Verification items for this drawing (mm, ordinates from the low corner). A direction names the side the tool comes from. Coordinates: 2 decimals unless noted, no trailing zeros. Order: outer loops, then holes, each group sorted by start corner. A loop starts at its lowest first (then second) coordinate and runs counter-clockwise, first axis right, second up. Notation, with made-up numbers: (82.25, 69) - (89.25, 69) arc R13 ccw to (89.25, 79) - close; hole circle Ø3 at (77, 8.5). An arc over 180 degrees is marked (long way). Use CSV: the item, a comma, the result in double quotes. Start each with the question number.
1) Tool access check on the marked faces 1 and 2. Record the directions out of +Z, -Z, +X, -X, +Y, -Y that give a thin tool (end or side, any length) a straight path to the whole face; none if there is none.
2) Sectioned sample at B-B, the plane x = 21. Record the cut outline in (y, z).
3) Thickness scan on probe 1 along X at (y, z) = (15.25, 4.5); probe 2 along Z at (x, y) = (17.75, 9.25); probe 3 along Z at (x, y) = (22.25, 10). Record the ranges inside material, lowest first. Write a range as [from, to].
4) Depth check by flat-ended pin: P1, Ø1.5, axis at x = 11, z = 4.5, coming from the +Y side; P2, Ø6, axis at x = 23.5, y = 15.5, coming from the +Z side; P3, Ø1, axis at y = 2, z = 8.5, coming from the +X side. Enter the tip coordinate at first touch or a pass-through.
5) Sectioned sample at A-A, the plane x = 5. Record the cut outline in (y, z) (1 decimal), and give its area (3 significant figures).
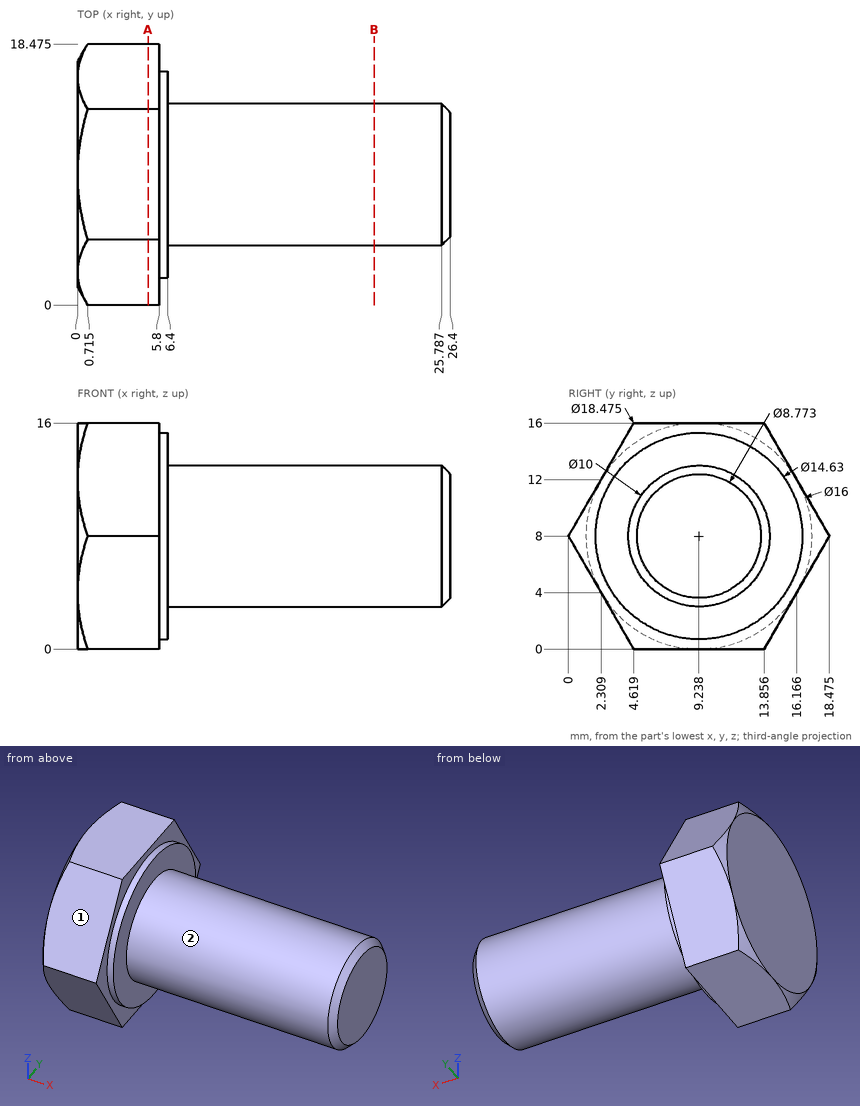
Evaluation:
1,face 1,"+Z, +X, -X, -Y"
1,face 2,"+X"
2,outline,"circle Ø10 at (9.24, 8)"
3,probe 1,"[0, 6.4]"
3,probe 2,"[3, 13]"
3,probe 3,"[3.06, 12.94]"
4,P1,"y = 13.41"
4,P2,"z = 11.79"
4,P3,"x = 6.4"
5,outline,"(0, 8) - (4.6, 0) - (13.9, 0) - (18.5, 8) - (13.9, 16) - (4.6, 16) - close"
5,area,"222 mm²"
